Part model, mm, in its own coordinate system. Face numbers are marked on the shaded views. Give positions to 0.01 mm unless a question says otherwise; leave off trailing zeros. Order: outer loops, then holes, each group sorted by start corner. A loop starts at its lowest first (then second) coordinate and runs counter-clockwise, first axis right, second up. Notation, with made-up numbers: (-26, 37) -> (3, 37) arc R10 ccw to (3, 56) -> close; hole circle Ø9 at (2.25, 59.25). An arc over 180 degrees is marked (long way). Write item = value, one per line. Start each with the question number.
(1) Saw through at D-D, the plane z = -53.5. List the corners of the cut face in (x, y).
(2) Saw through at C-C, the plane y = 31. State how many separate pieces and enclosed holes the cut face has, then the cut area to 3 significant figures.
(3) Saw through at A-A, the plane y = 7. List the corners of the cut face in (x, z).
(4) Flat gauge pins, fed straight in: pin 1 (3 mm diameter, centred on y = 17, z = -10.5, fed in from +X); pin 2 (10 mm diameter, centred on x = -81.5, z = -6.5, fed in from +Y); pin 3 (4 mm diameter, centred on y = 7, z = 55, fed in from +X); pin 4 (12 mm diameter, centred on y = 20.5, z = -13, fed in from -X). Where does each tip first touch, or does it go through?
(5) Saw through at B-B, the plane z = 70.5. List the corners of the cut face in (x, y).
(6) Two-plate mould, pull along Z, no slides. Class the marked faces 1, 2 and 3: pulls with the +Z half, pulls with the -Z half, needs draft (parallel to the pull), parting line crosses it, or undercut.
(7) Probe line 1 along Z through (x, y) = (0, 10.5); line 2 along Z through (x, y) = (0, 24.5); line 3 along Z through (x, y) = (17, 14). List the from-to ranges inside material, lowest first. Write a range as from..to.
from build123d import *

# Parameters (mm, degrees)
SKETCH1_R           = 106
BOSS_EXTRUDE1_DEPTH = 38
SKETCH2_R           = 100.2
SKETCH2_R_2         = 96.6
CUT_EXTRUDE1_DEPTH  = 36
SKETCH3_R           = 85.4
CUT_EXTRUDE2_DEPTH  = 155.647987378
SKETCH5_R           = 1.6
CUT_EXTRUDE3_DEPTH  = 155.647987378
CUT_EXTRUDE4_START  = -8
SKETCH6_R           = 1.6
CUT_EXTRUDE4_DEPTH  = 231.584815295
CIRPATTERN1_COUNT   = 4
CUT_EXTRUDE5_START  = 3
CUT_EXTRUDE5_DEPTH  = 2.8
CIRPATTERN2_COUNT   = 4


with BuildPart() as part:
    # Sketch1 → Boss-Extrude1 (new body)
    with BuildSketch(Plane(origin=(0, 0, 0), x_dir=(1, 0, 0), z_dir=(0, 1, 0))):
        with Locations(Location((0, 0, 0), (0, 0, 270))):
            Circle(SKETCH1_R)
    extrude(amount=BOSS_EXTRUDE1_DEPTH)

    # Sketch2 → Cut-Extrude1 (cut)
    with BuildSketch(Plane(origin=(0, 38, 0), x_dir=(1, 0, 0), z_dir=(0, 1, 0))):
        with Locations(Location((0, 0, 0), (0, 0, 270))):
            Circle(SKETCH2_R)
        with Locations(Location((0, 0, 0), (0, 0, 270))):
            Circle(SKETCH2_R_2, mode=Mode.SUBTRACT)
    extrude(amount=-CUT_EXTRUDE1_DEPTH, mode=Mode.SUBTRACT)

    # Sketch3 → Cut-Extrude2 (cut, through all)
    with BuildSketch(Plane(origin=(0, 38, 0), x_dir=(1, 0, 0), z_dir=(0, 1, 0))):
        with Locations(Location((0, 0, 0), (0, 0, 270))):
            Circle(SKETCH3_R)
    extrude(amount=-CUT_EXTRUDE2_DEPTH, mode=Mode.SUBTRACT)

    # Sketch5 → Cut-Extrude3 (cut, through all)
    with BuildSketch(Plane(origin=(0, 38, 0), x_dir=(1, 0, 0), z_dir=(0, 1, 0))):
        with Locations(Location((-64.346717088, 64.346717088, 0), (0, 0, 270))):
            Circle(SKETCH5_R)
        with Locations(Location((64.346717088, 64.346717088, 0), (0, 0, 270))):
            Circle(SKETCH5_R)
        with Locations(Location((64.346717088, -64.346717088, 0), (0, 0, 270))):
            Circle(SKETCH5_R)
        with Locations(Location((-64.346717088, -64.346717088, 0), (0, 0, 270))):
            Circle(SKETCH5_R)
    extrude(amount=-CUT_EXTRUDE3_DEPTH, mode=Mode.SUBTRACT)

    # Sketch6 → Cut-Extrude4 (cut)
    with BuildSketch(Plane.XY.offset(86).offset(CUT_EXTRUDE4_START)):
        with Locations(Location((0, 16, 0), (0, 0, 270))):
            Circle(SKETCH6_R)
    cut_extrude4 = extrude(amount=CUT_EXTRUDE4_DEPTH, mode=Mode.SUBTRACT)

    # CirPattern1: Cut-Extrude4 ×4 about axis
    cirpattern1_axis = Axis((0, 38, 0), (0, -1, 0))
    for i in range(1, CIRPATTERN1_COUNT):
        add(cut_extrude4.rotate(cirpattern1_axis, i * 360 / CIRPATTERN1_COUNT), mode=Mode.SUBTRACT)

    # Sketch7 → Cut-Extrude5 (cut)
    with BuildSketch(Plane.XY.offset(86).offset(CUT_EXTRUDE5_START)):
        Polygon((-3.05, 17.760918321), (-3.05, 37.760918321), (3.05, 37.760918321), (3.05, 17.760918321), (3.05, 14.239081679), (0, 12.478163358), (-3.05, 14.239081679), align=None)
    cut_extrude5 = extrude(amount=CUT_EXTRUDE5_DEPTH, mode=Mode.SUBTRACT)

    # CirPattern2: Cut-Extrude5 ×4 about axis
    cirpattern2_axis = Axis((0, 0, 0), (0, 1, 0))
    for i in range(1, CIRPATTERN2_COUNT):
        add(cut_extrude5.rotate(cirpattern2_axis, i * 360 / CIRPATTERN2_COUNT), mode=Mode.SUBTRACT)


solid = part.part
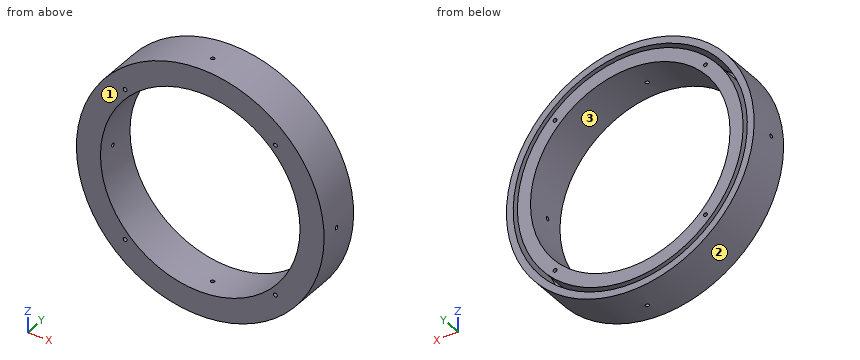
Results list:
q1.outline = (-91.51, 0) -> (-66.57, 0) -> (-66.57, 38) -> (-80.43, 38) -> (-80.43, 2) -> (-84.72, 2) -> (-84.72, 38) -> (-91.51, 38) -> close; (66.57, 0) -> (91.51, 0) -> (91.51, 38) -> (84.72, 38) -> (84.72, 2) -> (80.43, 2) -> (80.43, 38) -> (66.57, 38) -> close
q2.separate_pieces = 2
q2.enclosed_holes = 10
q2.area = 10,100 mm^2
q3.outline = circle Ø212 at (0, 0); circle Ø193.2 at (0, 0); hole circle Ø200.4 at (0, 0); hole circle Ø170.8 at (0, 0); hole circle Ø3.2 at (-64.35, -64.35); hole circle Ø3.2 at (-64.35, 64.35); hole circle Ø3.2 at (64.35, -64.35); hole circle Ø3.2 at (64.35, 64.35)
q4.pin_1 = 105.62
q4.pin_2 = 38
q4.pin_3 = 91.8
q4.pin_4 = -105.77
q5.outline = (-79.16, 0) -> (-48.2, 0) -> (-48.2, 38) -> (-66.04, 38) -> (-66.04, 2) -> (-71.2, 2) -> (-71.2, 38) -> (-79.16, 38) -> close; (48.2, 0) -> (79.16, 0) -> (79.16, 38) -> (71.2, 38) -> (71.2, 2) -> (66.04, 2) -> (66.04, 38) -> (48.2, 38) -> close
q6.face_1 = needs draft
q6.face_2 = parting line crosses it
q6.face_3 = undercut
q7.line_1 = -106..-100.2, -96.6..-85.4, 85.4..96.6, 100.2..106
q7.line_2 = -106..-100.2, -96.6..-91.8, -89..-85.4, 85.4..89, 91.8..96.6, 100.2..106
q7.line_3 = -104.63..-98.75, -95.09..-83.69, 83.69..95.09, 98.75..104.63
